Verification items for the finished model (mm, model axes). Face numbers are marked on the shaded views. A direction names the side the tool comes from. Coordinates: 2 decimals unless noted, no trailing zeros. Order: outer loops, then holes, each group sorted by start corner. A loop starts at its lowest first (then second) coordinate and runs counter-clockwise, first axis right, second up. Notation, with made-up numbers: M 73,-19.5 L 123,-19.5 A27 ccw 123,-0.5 Z; hole C -3.75,4.25 d9. An arc over 180 degrees is marked long. Return JSON: item names as keys, results as strings. Group by question number.
1. Section check D-D, the plane x = 22.5. Record the cut outline in (y, z), plus the area to 3 significant figures.
2. Gauge pin test, flat ends, axial feed: pin 1 (1.5 mm diameter, centred on x = 5, z = 16, fed in from -Y); pin 2 (1 mm diameter, centred on y = 3, z = 36.5, fed in from +X); pin 3 (0.9 mm diameter, centred on y = 15, z = 42.5, fed in from +X); pin 4 (2 mm diameter, centred on y = 8.5, z = 22.5, fed in from +X). Record the tip position at first contact, or that the pin passes through.
3. Mould release check, pull along Z, two halves, no side actions. Record for the marked faces 3, 4 and 5: +Z half, -Z half, draft (parallel to the pull), parting line (faces both ways), or undercut.
4. Material ranges on line 1 along Z through (x, y) = (10.5, 15.75); line 2 along Z through (x, y) = (22.75, 15.75); line 3 along Y through (x, z) = (3, 34.5), recorded low to high.
5. Section check B-B, the plane y = 6. Record the cut outline in (x, z), plus the area to 3 significant figures.
6. Set-up check for the marked faces 1 and 2: record each of +Z, -Z, +X, -X, +Y, -Y from which the full face is reachable in a straight line by a thin tool's end or side.
7. Section check C-C, the plane z = 31. Record the cut outline in (x, y).
8. Section check A-A, the plane x = 26.25. Record the cut outline in (y, z).
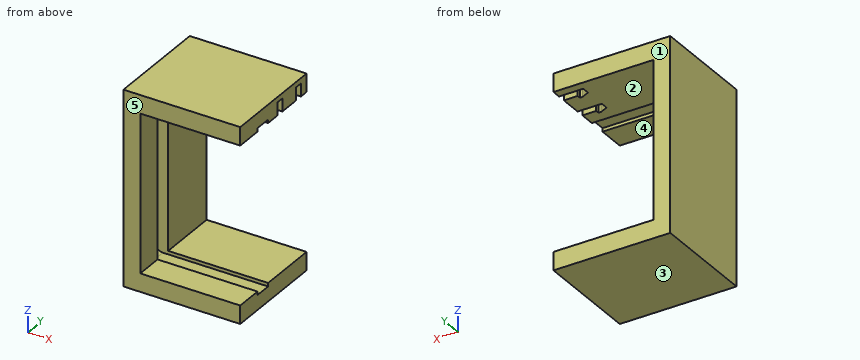
```python
from build123d import *

# Parameters (mm, degrees)
SKETCH1_W           = 4
SKETCH1_H           = 25
BOSS_EXTRUDE1_DEPTH = 46
BOSS_EXTRUDE2_START = -25
BOSS_EXTRUDE2_DEPTH = 25
CAVITY2_START       = 6.511576254
CAVITY2_DEPTH       = 4
CUT_EXTRUDE6_START  = -25
SKETCH8_W           = 23.75
SKETCH8_H           = 0.48
CUT_EXTRUDE6_DEPTH  = 25
SKETCH10_W          = 0.5
SKETCH10_H          = 4
CUT_EXTRUDE8_DEPTH  = 25
CUT_EXTRUDE9_DEPTH  = 4.322904331
BOSS_EXTRUDE4_DEPTH = 1.25
SKETCH13_W          = 0.15
SKETCH13_H          = 0.85
CUT_EXTRUDE10_DEPTH = 3.072904331
LPATTERN4_COUNT     = 2
LPATTERN4_PITCH     = 7


# Read off the part's stored shape, not the designer's step: Cavity2
with BuildPart() as part:
    # Sketch1 → Boss-Extrude1 (new body)
    with BuildSketch(Plane.XY):
        with Locations((2, 12.5)):
            Rectangle(SKETCH1_W, SKETCH1_H)
    extrude(amount=BOSS_EXTRUDE1_DEPTH)

    # Sketch2 → Boss-Extrude2 (add)
    with BuildSketch(Plane(origin=(0, 25, 0), x_dir=(1, 0, 0), z_dir=(0, 1, 0)).offset(BOSS_EXTRUDE2_START)):
        Polygon((27.75, -3.5), (27.75, -4.318971826), (4, -4.318971826), (4, -3.5), (4, 0), (27.75, 0), align=None)
        Polygon((4, -46), (27.75, -46), (27.75, -42), (27.75, -41.197095669), (4, -41.197095669), (4, -42), align=None)
    extrude(amount=BOSS_EXTRUDE2_DEPTH)

    # Cavity2 outline → Cavity2 (cut)
    with BuildSketch(Plane(origin=(0, 0, 0), x_dir=(1, 0, 0), z_dir=(0, 1, 0)).offset(CAVITY2_START)):
        with BuildLine():
            Line((1, -5.25), (1, -40.25))
            ThreePointArc((1, -40.25), (1.512563133, -41.487436867), (2.75, -42))
            Line((2.75, -42), (27.75, -42))
            Line((27.75, -42), (27.75, -41.197095669))
            Line((27.75, -41.197095669), (4, -41.197095669))
            Line((4, -41.197095669), (4, -4.318971826))
            Line((4, -4.318971826), (27.75, -4.318971826))
            Line((27.75, -4.318971826), (27.75, -3.5))
            Line((27.75, -3.5), (2.75, -3.5))
            ThreePointArc((2.75, -3.5), (1.512563133, -4.012563133), (1, -5.25))
        make_face()
    extrude(amount=CAVITY2_DEPTH, mode=Mode.SUBTRACT)

    # Sketch8 → Cut-Extrude6 (cut)
    with BuildSketch(Plane(origin=(0, 25, 0), x_dir=(1, 0, 0), z_dir=(0, 1, 0)).offset(CUT_EXTRUDE6_START)):
        with Locations((15.875, -41.437095669)):
            Rectangle(SKETCH8_W, SKETCH8_H)
    extrude(amount=CUT_EXTRUDE6_DEPTH, mode=Mode.SUBTRACT)

    # Sketch10 → Cut-Extrude8 (cut)
    with BuildSketch(Plane(origin=(27.75, 0, 0), x_dir=(0, 0, -1), z_dir=(1, 0, 0))):
        with Locations((-42.25, 8.511576254)):
            Rectangle(SKETCH10_W, SKETCH10_H)
    extrude(amount=-CUT_EXTRUDE8_DEPTH, mode=Mode.SUBTRACT)

    # Sketch11 → Cut-Extrude9 (cut)
    with BuildSketch(Plane.XY.offset(46)):
        Polygon((22, 22.9), (22, 21.1), (23.86, 20.25), (24.31, 20.25), (24.31, 21.1), (27.75, 21.1), (27.75, 22.9), (24.352614362, 22.9), align=None)
    cut_extrude9 = extrude(amount=-CUT_EXTRUDE9_DEPTH, mode=Mode.SUBTRACT)

    # Sketch12 → Boss-Extrude4 (add)
    with BuildSketch(Plane.XY.offset(46)):
        Polygon((27.75, 21.1), (27.75, 22.9), (22, 22.9), (22, 21.1), (23.86, 20.25), (24.31, 20.25), (24.31, 21.1), align=None)
    boss_extrude4 = extrude(amount=-BOSS_EXTRUDE4_DEPTH)

    # Sketch13 → Cut-Extrude10 (cut)
    with BuildSketch(Plane(origin=(0, 0, 41.677095669), x_dir=(-1, 0, 0), z_dir=(0, 0, -1))):
        with Locations((-24.385, 20.675)):
            Rectangle(SKETCH13_W, SKETCH13_H)
    cut_extrude10 = extrude(amount=-CUT_EXTRUDE10_DEPTH, mode=Mode.SUBTRACT)

    # LPattern4: Cut-Extrude9, Boss-Extrude4, Cut-Extrude10 ×2
    with Locations(*[(0, -i * LPATTERN4_PITCH, 0) for i in range(1, LPATTERN4_COUNT)]):
        add(cut_extrude9, mode=Mode.SUBTRACT)
        add(boss_extrude4)
        add(cut_extrude10, mode=Mode.SUBTRACT)


solid = part.part
```
Answers follow:
{
 "1": {"outline": "M 0,0 L 25,0 L 25,4.32 L 10.51,4.32 L 10.51,3.5 L 6.51,3.5 L 6.51,4.32 L 0,4.32 Z; M 0,41.68 L 6.51,41.68 L 6.51,42.5 L 10.51,42.5 L 10.51,41.68 L 13.87,41.68 L 13.87,44.75 L 15.9,44.75 L 15.9,41.68 L 20.87,41.68 L 20.87,44.75 L 22.9,44.75 L 22.9,41.68 L 25,41.68 L 25,46 L 0,46 Z", "area": "197 mm^2"},
 "2": {"pin 1": "through", "pin 2": "x = 4", "pin 3": "x = 22", "pin 4": "x = 1"},
 "3": {"face 3": "-Z half", "face 4": "undercut", "face 5": "draft"},
 "4": {"line 1": "0 to 4.32, 41.68 to 46", "line 2": "0 to 4.32, 44.75 to 46", "line 3": "0 to 6.51, 10.51 to 25"},
 "5": {"outline": "M 0,0 L 27.75,0 L 27.75,4.32 L 4,4.32 L 4,41.68 L 27.75,41.68 L 27.75,46 L 0,46 Z", "area": "389 mm^2"},
 "6": {"face 1": "+Z, -Z, +X, -X, +Y", "face 2": "+X, +Y, -Y"},
 "7": {"outline": "M 0,0 L 4,0 L 4,6.51 L 1,6.51 L 1,10.51 L 4,10.51 L 4,25 L 0,25 Z"},
 "8": {"outline": "M 0,0 L 25,0 L 25,4.32 L 10.51,4.32 L 10.51,3.5 L 6.51,3.5 L 6.51,4.32 L 0,4.32 Z; M 0,41.68 L 6.51,41.68 L 6.51,42.5 L 10.51,42.5 L 10.51,41.68 L 14.1,41.68 L 14.1,44.75 L 15.9,44.75 L 15.9,41.68 L 21.1,41.68 L 21.1,44.75 L 22.9,44.75 L 22.9,41.68 L 25,41.68 L 25,46 L 0,46 Z"}
}
